```python
from build123d import *

# Parameters (mm, degrees)
SKETCH1_W      = 150
SKETCH1_H      = 160
EXTRUDE1_DEPTH = 20
EXTRUDE2_DEPTH = 30
EXTRUDE3_DEPTH = 50
EXTRUDE4_DEPTH = 161
SKETCH5_R      = 127.5
EXTRUDE5_DEPTH = 0.01


with BuildPart() as part:
    # Sketch1 → Extrude1 (new body)
    with BuildSketch(Plane(origin=(0, 0, 0), x_dir=(1, 0, 0), z_dir=(0, 1, 0))):
        with Locations((75, 80)):
            Rectangle(SKETCH1_W, SKETCH1_H)
    extrude(amount=EXTRUDE1_DEPTH)

    # Sketch2 → Extrude2 (add)
    with BuildSketch(Plane(origin=(0, 20, 0), x_dir=(1, 0, 0), z_dir=(0, 1, 0))):
        Polygon((75, 140), (23.038475773, 110), (23.038475773, 50), (75, 20), (126.961524227, 50), (126.961524227, 110), align=None)
    extrude(amount=EXTRUDE2_DEPTH)

    # Sketch3 → Extrude3 (add)
    with BuildSketch(Plane(origin=(0, 50, 0), x_dir=(1, 0, 0), z_dir=(0, 1, 0))):
        Polygon((40, 90), (40, 70), (90, 80), align=None)
    extrude(amount=EXTRUDE3_DEPTH)

    # Sketch4 → Extrude4 (cut, through all)
    with BuildSketch(Plane.XY):
        with BuildLine():
            Line((110, 95), (110, 50))
            Line((110, 50), (65, 50))
            ThreePointArc((65, 50), (78.180194847, 81.819805153), (110, 95))
        make_face()
        Polygon((40, 50), (90, 100), (40, 100), align=None)
    extrude(amount=-EXTRUDE4_DEPTH, mode=Mode.SUBTRACT)

    # Sketch5 → Extrude5 (add)
    with BuildSketch(Plane(origin=(0, 0, 0), x_dir=(1, 0, 0), z_dir=(0, 1, 0))):
        with Locations(Location((75, 80, 0), (0, 0, 270))):  # turned: the seam where the file's is
            Circle(SKETCH5_R)
    extrude(amount=EXTRUDE5_DEPTH)


solid = part.part
```
Check sheet for the modelled part. Datum: model origin and axes. Units: mm. A direction names the side the tool comes from. Coordinates: 2 decimals unless noted, no trailing zeros. Order: outer loops, then holes, each group sorted by start corner. A loop starts at its lowest first (then second) coordinate and runs counter-clockwise, first axis right, second up. Notation, with made-up numbers: (-35, 60) -> (14, 60) arc R25 cw to (14, 95) -> close; hole circle Ø3 at (57, -15). An arc over 180 degrees is marked (long way). Write item = value, one per line. Start each with the question number.
1) Material ranges on L1, parallel to Z at x = 13.5, y = 7; L2, parallel to Y at x = 25, z = -44.5; L3, parallel to Y at x = 72, z = -58, recorded low to high.
2) Access from +Z, -Z, +X, -X, +Y, -Y to the whole of each face (thin tool, end or side, straight path). Record for faces 5 (the flat face through (101.344, 34.79, -124.79)), 6 (the flat face through (100.62, 34.79, -34.79)), 7 (the flat face through (126.962, 35, -80)).
3) Mould release check, pull along Y, two halves, no side actions. Record for faces 1 (the cylindrical face through (68.985, 68.513, -79.93)), 2 (the flat face through (91, 20, -134)), 3 (the flat face through (65, 67, -75)), 4 (the flat face through (77, 0, -82)): +Y half, -Y half, draft (parallel to the pull), parting line (faces both ways), or undercut.
4) Cross-section at A-A (y = 24). Enter the section's corners in (x, z), then the cut area to 3 significant figures.
5) Go/stop test with flat-tipped pins: P1, Ø1.5, axis at x = 117.5, y = 52, coming from the -Z side; P2, Ø22, axis at y = 14.5, z = -99, coming from the +X side; P3, Ø2, axis at x = 11, z = -145.5, coming from the +Y side; P4, Ø6, axis at x = 40, y = 7, coming from the +Z side. Record where each tip stops, or that it passes through.
Ans:
q1.L1 = -160 to 0
q1.L2 = 0 to 20
q1.L3 = 0 to 50
q2.face_5 = -Z, +X, +Y
q2.face_6 = +Z, +X, +Y
q2.face_7 = +Z, -Z, +X, +Y
q3.face_1 = undercut
q3.face_2 = +Y half
q3.face_3 = draft
q3.face_4 = -Y half
q4.outline = (23.04, -110) -> (75, -140) -> (126.96, -110) -> (126.96, -50) -> (75, -20) -> (23.04, -50) -> close
q4.area = 9,350 mm²
q5.P1 = through
q5.P2 = 150
q5.P3 = 20
q5.P4 = 0
